from build123d import *

# Parameters (mm, degrees)
SKETCH1_R           = 2
BOSS_EXTRUDE1_DEPTH = 8.5
SKETCH9_W           = 8.5
SKETCH9_H           = 5
BOSS_EXTRUDE4_DEPTH = 4
SKETCH6_W           = 7
SKETCH6_H           = 1.6
CUT_EXTRUDE5_DEPTH  = 20.931131428
BOSS_EXTRUDE3_DEPTH = 7
SKETCH10_W          = 5
SKETCH10_H          = 1
CUT_EXTRUDE6_DEPTH  = 19.607794066


with BuildPart() as part:
    # Sketch1 → Boss-Extrude1 (new body)
    with BuildSketch(Plane.XY):
        with BuildLine():
            Line((-3, 0), (-3, -12))
            ThreePointArc((-3, -12), (0, -15), (3, -12))
            Line((3, -12), (3, 0))
            ThreePointArc((3, 0), (0, 3), (-3, 0))
        make_face()
        Circle(SKETCH1_R, mode=Mode.SUBTRACT)
        with Locations((0, -12)):
            Circle(SKETCH1_R, mode=Mode.SUBTRACT)
    extrude(amount=BOSS_EXTRUDE1_DEPTH)

    # Sketch9 → Boss-Extrude4 (add)
    with BuildSketch(Plane.ZY.offset(3)):
        with Locations((4.25, -5.5)):
            Rectangle(SKETCH9_W, SKETCH9_H)
    extrude(amount=BOSS_EXTRUDE4_DEPTH)

    # Sketch6 → Cut-Extrude5 (cut, through all)
    with BuildSketch(Plane(origin=(3, 0, 0), x_dir=(0, 0, -1), z_dir=(1, 0, 0))):
        with Locations((-3.5, -5.3)):
            Rectangle(SKETCH6_W, SKETCH6_H)
    extrude(amount=-CUT_EXTRUDE5_DEPTH, mode=Mode.SUBTRACT)

    # Sketch7 → Boss-Extrude3 (add, through all)
    with BuildSketch(Plane(origin=(0, 0, 7), x_dir=(-1, 0, 0), z_dir=(0, 0, -1))):
        with BuildLine():
            Line((-3, -6.1), (-3, -5.5))
            ThreePointArc((-3, -5.5), (-2.956066017, -5.393933983), (-2.85, -5.35))
            Line((-2.85, -5.35), (-2.15, -5.35))
            ThreePointArc((-2.15, -5.35), (-2.043933983, -5.393933983), (-2, -5.5))
            Line((-2, -5.5), (-2, -6.1))
            Line((-2, -6.1), (-3, -6.1))
        make_face()
        with BuildLine():
            Line((-0.85, -5.35), (-0.15, -5.35))
            ThreePointArc((-0.15, -5.35), (-0.043933983, -5.393933983), (0, -5.5))
            Line((0, -5.5), (0, -6.1))
            Line((0, -6.1), (-1, -6.1))
            Line((-1, -6.1), (-1, -5.5))
            ThreePointArc((-1, -5.5), (-0.956066017, -5.393933983), (-0.85, -5.35))
        make_face()
        with BuildLine():
            Line((1.15, -5.35), (1.85, -5.35))
            ThreePointArc((1.85, -5.35), (1.956066017, -5.393933983), (2, -5.5))
            Line((2, -5.5), (2, -6.1))
            Line((2, -6.1), (1, -6.1))
            Line((1, -6.1), (1, -5.5))
            ThreePointArc((1, -5.5), (1.043933983, -5.393933983), (1.15, -5.35))
        make_face()
        with BuildLine():
            Line((3.15, -5.35), (3.85, -5.35))
            ThreePointArc((3.85, -5.35), (3.956066017, -5.393933983), (4, -5.5))
            Line((4, -5.5), (4, -6.1))
            Line((4, -6.1), (3, -6.1))
            Line((3, -6.1), (3, -5.5))
            ThreePointArc((3, -5.5), (3.043933983, -5.393933983), (3.15, -5.35))
        make_face()
        with BuildLine():
            Line((5.15, -5.35), (5.85, -5.35))
            ThreePointArc((5.85, -5.35), (5.956066017, -5.393933983), (6, -5.5))
            Line((6, -5.5), (6, -6.1))
            Line((6, -6.1), (5, -6.1))
            Line((5, -6.1), (5, -5.5))
            ThreePointArc((5, -5.5), (5.043933983, -5.393933983), (5.15, -5.35))
        make_face()
    extrude(amount=BOSS_EXTRUDE3_DEPTH)

    # Sketch10 → Cut-Extrude6 (cut, through all)
    with BuildSketch(Plane.XY.offset(8.5)):
        with Locations((0, 3)):
            Rectangle(SKETCH10_W, SKETCH10_H)
    extrude(amount=-CUT_EXTRUDE6_DEPTH, mode=Mode.SUBTRACT)


solid = part.part
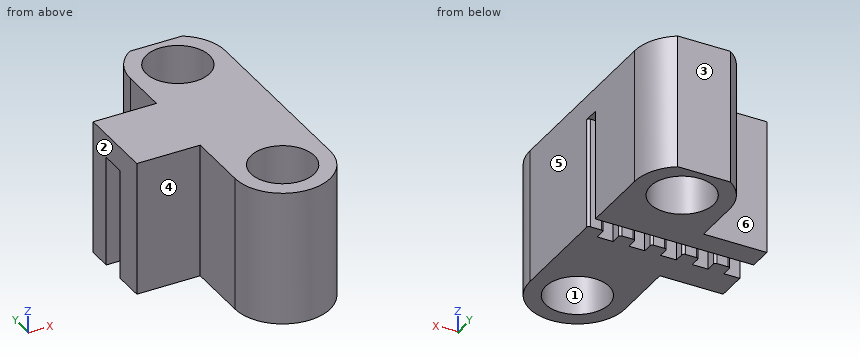
Verification items for the finished model (mm, model axes). Face numbers are marked on the shaded views. A direction names the side the tool comes from. Coordinates: 2 decimals unless noted, no trailing zeros. Order: outer loops, then holes, each group sorted by start corner. A loop starts at its lowest first (then second) coordinate and runs counter-clockwise, first axis right, second up. Notation, with made-up numbers: (-2, 66.5) -> (10, 66.5) arc R27 ccw to (10, 101.5) -> close; hole circle Ø3 at (67.5, 42). An arc over 180 degrees is marked (long way). Use CSV: the item, a comma, the result in double quotes. Start each with the question number.
Q1. Tool access check on the marked faces 4, 5 and 6. Record the directions out of +Z, -Z, +X, -X, +Y, -Y that give a thin tool (end or side, any length) a straight path to the whole face; none if there is none.
Q2. Thickness scan on line 1 along Y through (x, z) = (-0.5, 2.75); line 2 along Y through (x, z) = (0.25, 4); line 3 along Y through (x, z) = (-4.25, 2.5). Record the ranges inside material, lowest first.
Q3. Draft check along X on the marked faces 1, 2 and 3. Enter one of: +X half, -X half, draft (parallel to the pull), parting line (faces both ways), or undercut.
Q4. Section check A-A, the plane y = -12.5. Record the cut outline in (x, z).
Q5. Section check C-C, the plane z = 4. Give the number of separate pieces and of enclosed holes in the cut face, and give its area (3 significant figures).
Q6. Depth check by flat-ended pin: P1, Ø1, axis at x = -2.5, z = 7.5, coming from the +Y side; P2, Ø1.2, axis at x = -6, z = 5, coming from the -Y side; P3, Ø1.5, axis at y = -1, z = 3, coming from the -X side. Enter the tip coordinate at first touch or a pass-through.
Q7. Section check B-B, the plane z = 7.75. Record the cut outline in (x, y).
Q8. Section check D-D, the plane y = -5. Record the cut outline in (x, z).
Returned:
1,face 4,"+Z, -Z, -X, -Y"
1,face 5,"+Z, -Z, +X, +Y, -Y"
1,face 6,"+Z, -Z, -X, +Y"
2,line 1,"y = -14.96 to -13.94, -10.06 to -6.1, -4.5 to -1.94, 1.94 to 2.5"
2,line 2,"y = -14.99 to -13.98, -10.02 to -5.35, -4.5 to -1.98, 1.98 to 2.5"
2,line 3,"y = -8 to -6.1, -4.5 to -3"
3,face 1,"undercut"
3,face 2,"-X half"
3,face 3,"draft"
4,outline,"(-2.96, 0) -> (-1.94, 0) -> (-1.94, 8.5) -> (-2.96, 8.5) -> close; (1.94, 0) -> (2.96, 0) -> (2.96, 8.5) -> (1.94, 8.5) -> close"
5,separate pieces,"2"
5,enclosed holes,"2"
5,area,"81.7 mm^2"
6,P1,"stops at y = 2.24"
6,P2,"stops at y = -8"
6,P3,"stops at x = -3"
7,outline,"(-7, -8) -> (-3, -8) -> (-3, -12) arc R3 ccw to (3, -12) -> (3, 0) arc R3 ccw to (1.66, 2.5) -> (-1.66, 2.5) arc R3 ccw to (-3, 0) -> (-3, -3) -> (-7, -3) -> close; hole circle Ø4 at (0, -12); hole circle Ø4 at (0, 0)"
8,outline,"(-7, 7) -> (3, 7) -> (3, 8.5) -> (-7, 8.5) -> close"
